Geometry: final body of the model. Coordinates: model frame, mm. Give positions to 0.01 mm unless a question says otherwise; leave off trailing zeros. Order: outer loops, then holes, each group sorted by start corner. A loop starts at its lowest first (then second) coordinate and runs counter-clockwise, first axis right, second up. Notation, with made-up numbers: (-24, 56) - (2, 56) arc R17 cw to (2, 84) - close; hole circle Ø3 at (-24, 47). An arc over 180 degrees is marked (long way). Use one line per item in the form item = value.
from build123d import *

# Parameters (mm, degrees)
F1_DEPTH = 6.35
F3_D     = 12.7


with BuildPart() as f1:
    # F0 (on Front) → F1 (new body)
    with BuildSketch(Plane.XZ):
        Polygon((20.06367, 44.286881), (0, 51.137887), (0, 0), align=None)
        Polygon((0, 0), (0, 51.137887), (-17.616881, 44.286881), align=None)
        Polygon((20.06367, 44.286881), (0, 0), (38.169909, 30.584864), align=None)
        Polygon((38.169909, 30.584864), (0, 0), (46.978351, 11.25523), align=None)
        Polygon((46.978351, 11.25523), (0, 0), (46.978351, 0), align=None)
        Polygon((-34.716997, 30.584864), (0, 0), (-17.616881, 44.286881), align=None)
        Polygon((-42.818807, 11.25523), (0, 0), (-34.716997, 30.584864), align=None)
        Polygon((-42.818807, 0), (0, 0), (-42.818807, 11.25523), align=None)
    extrude(amount=F1_DEPTH)

    # F3 (through all)
    with Locations(Plane(origin=(0, 0, 0), x_dir=(1, 0, 0), z_dir=(0, 1, 0))):
        with Locations((0, 0)):
            Hole(F3_D / 2)


solid = f1.part
(1) Pull-direction query (X, two-part tool) for faces 1 (the face through (46.978, -3, 6)), 2 (the face through (-25, -3, 0)), 3 (the face through (0.14, -3.22, 6.35)); classes: released by +X, released by -X, zero draft, split by the parting line, or undercut.
Computed values:
face_1 = released by +X
face_2 = zero draft
face_3 = undercut
(2) Cut plane A-A on y = -1.25. Output: boundary loops of the cut face in (x, z), plus the area to 3 significant figures.
Computed values:
outline = (-42.82, 0) - (-6.35, 0) arc R6.35 cw to (6.35, 0) - (46.98, 0) - (46.98, 11.26) - (38.17, 30.58) - (20.06, 44.29) - (0, 51.14) - (-17.62, 44.29) - (-34.72, 30.58) - (-42.82, 11.26) - close
area = 3,410 mm²
(3) Ray query, line 1 along Z through (x, y) = (-30.5, -0.5); line 2 along Z through (x, y) = (37.5, -2.5); line 3 along X through (y, z) = (-1, 17.5). Return the intervals inside material, ascending.
Computed values:
line_1 = 0 to 33.96
line_2 = 0 to 31.09
line_3 = -40.2 to 44.13
(4) Cut plane C-C on x = 12. Output: boundary loops of the cut face in (y, z), plus the area to 3 significant figures.
Computed values:
outline = (-6.35, 0) - (0, 0) - (0, 47.04) - (-6.35, 47.04) - close
area = 299 mm²
(5) Contact query for flat-ended pins moving along their axis: pin 1 Ø2 at (y, z) = (-5, 14.5) entering from -X; pin 2 Ø1.5 at (x, y) = (-33.5, -4) entering from +Z. Output: stop coordinate, or through.
Computed values:
pin_1 = -41.88
pin_2 = 32.16
(6) Cut plane B-B on z = 13.5. Output: boundary loops of the cut face in (x, y), plus the area to 3 significant figures.
Computed values:
outline = (-41.88, -6.35) - (45.96, -6.35) - (45.96, 0) - (-41.88, 0) - close
area = 558 mm²
